Can you work these out from the drawing? Everything is in mm from the part's minimum corner. Coordinates: 2 decimals unless noted, no trailing zeros. Order: outer loops, then holes, each group sorted by start corner. A loop starts at its lowest first (then second) coordinate and runs counter-clockwise, first axis right, second up. Notation, with made-up numbers: (68.25, -12) -> (105.25, -12) arc R30 ccw to (105.25, 23) -> close; hole circle Ø5 at (45, -1). An arc over 180 degrees is marked (long way). Return JSON: item names as keys, results as strings. Group by question number.
1) For pin 1 (5 mm diameter, centred on y = 18, z = 9, fed in from +X); pin 2 (1 mm diameter, centred on x = 112.5, z = 6, fed in from -Y); pin 3 (3 mm diameter, centred on x = 31.5, z = 4, fed in from -Y), each with a flat end and sliding along its axis, tell me the tip position at first contact or that it passes through.
2) If I drill on probe 1 along Y at (x, z) = (15, 3.5); probe 2 along X at (y, z) = (17, 2.25); probe 3 along Y at (x, z) = (29, 6.5), over which ranges is the centre line in solid material (lowest first)? Write a range as from..to.
3) If we section it at C-C, the plane z = 4: Please give me the cut outline in (x, y), then the cut area to 3 significant figures.
4) If we section it at B-B, the plane y = 30: Please give me the cut outline in (x, z), then the cut area to 3 significant figures.
5) If we section it at D-D, the plane y = 70: Please give me the cut outline in (x, z).
6) If we section it at A-A, the plane x = 15: Please give me the cut outline in (y, z), then the cut area to 3 significant figures.
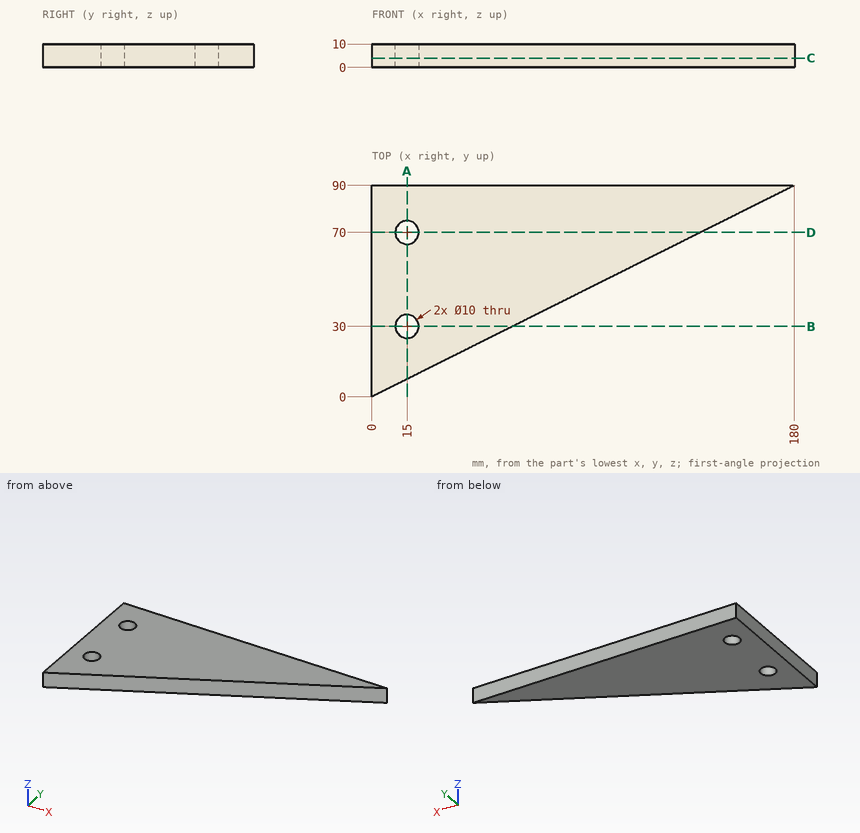
Result sheet:
{
 "1": {"pin 1": "stops at x = 41", "pin 2": "stops at y = 56", "pin 3": "stops at y = 15"},
 "2": {"probe 1": "y = 7.5..25, 35..65, 75..90", "probe 2": "x = 0..34", "probe 3": "y = 14.5..90"},
 "3": {"outline": "(0, 0) -> (180, 90) -> (0, 90) -> close; hole circle Ø10 at (15, 30); hole circle Ø10 at (15, 70)", "area": "7,940 mm2"},
 "4": {"outline": "(0, 0) -> (10, 0) -> (10, 10) -> (0, 10) -> close; (20, 0) -> (60, 0) -> (60, 10) -> (20, 10) -> close", "area": "500 mm2"},
 "5": {"outline": "(0, 0) -> (10, 0) -> (10, 10) -> (0, 10) -> close; (20, 0) -> (140, 0) -> (140, 10) -> (20, 10) -> close"},
 "6": {"outline": "(7.5, 0) -> (25, 0) -> (25, 10) -> (7.5, 10) -> close; (35, 0) -> (65, 0) -> (65, 10) -> (35, 10) -> close; (75, 0) -> (90, 0) -> (90, 10) -> (75, 10) -> close", "area": "625 mm2"}
}
